```python
from build123d import *

# Parameters (mm, degrees)
F0_W     = 85
F0_H     = 56
F0_R     = 1.375
F1_DEPTH = 1.5
F2_W     = 14.5066131875
F2_H     = 7.0550842881
F2_H_2   = 1.0795340971
F3_DEPTH = 4
F2_W_2   = 52.5494457505
F2_H_3   = 3.6331438509
F4_DEPTH = 9
F2_W_3   = 0.706913475
F2_H_4   = 12.0032178172
F2_W_4   = 17.4915134945
F2_W_5   = 0.87367237
F2_W_6   = 17.3247545996
F5_DEPTH = 15
F2_W_7   = 20.1837714718
F2_H_5   = 16.9899400229
F2_W_8   = 1.3980423616
F6_DEPTH = 13


with BuildPart() as f1:
    # F0 (on Top) → F1 (new body)
    with BuildSketch(Plane.XY):
        Rectangle(F0_W, F0_H)
        with Locations((-39, -24.5)):
            Circle(F0_R, mode=Mode.SUBTRACT)
        with Locations((19, -24.5)):
            Circle(F0_R, mode=Mode.SUBTRACT)
        with Locations((-39, 24.5)):
            Circle(F0_R, mode=Mode.SUBTRACT)
        with Locations((19, 24.5)):
            Circle(F0_R, mode=Mode.SUBTRACT)
    extrude(amount=F1_DEPTH)

    # F2 (on face) → F3 (join)
    with BuildSketch(Plane.XY.offset(1.5)):
        with Locations((-10.5, -24.4724578559)):
            Rectangle(F2_W, F2_H)
        with Locations((-10.5, -28.5397670486)):
            Rectangle(F2_W, F2_H_2)
    extrude(amount=F3_DEPTH)

    # F2 (on face) → F4 (join)
    with BuildSketch(Plane.XY.offset(1.5)):
        with Locations((-9.9811840151, 23.979865989)):
            Rectangle(F2_W_2, F2_H_3)
    extrude(amount=F4_DEPTH)

    # F2 (on face) → F5 (join)
    with BuildSketch(Plane.XY.offset(1.5)):
        with Locations((42.8534567375, 3.2353831921)):
            Rectangle(F2_W_3, F2_H_4)
        with Locations((33.7542432528, 3.2353831921)):
            Rectangle(F2_W_4, F2_H_4)
        with Locations((42.936836185, 19.5779297501)):
            Rectangle(F2_W_5, F2_H_4)
        with Locations((33.8376227002, 19.5779297501)):
            Rectangle(F2_W_6, F2_H_4)
    extrude(amount=F5_DEPTH)

    # F2 (on face) → F6 (join)
    with BuildSketch(Plane.XY.offset(1.5)):
        with Locations((32.4081142641, -15.4418135062)):
            Rectangle(F2_W_7, F2_H_5)
        with Locations((43.1990211808, -15.4418135062)):
            Rectangle(F2_W_8, F2_H_5)
    extrude(amount=F6_DEPTH)


solid = f1.part
```
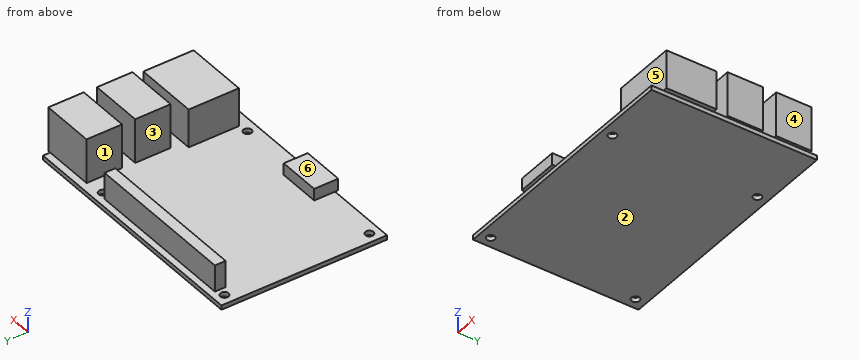
Part model, mm, in its own coordinate system. Face numbers are marked on the shaded views. A direction names the side the tool comes from. Give positions to 0.01 mm unless a question says otherwise; leave off trailing zeros. Order: outer loops, then holes, each group sorted by start corner. A loop starts at its lowest first (then second) coordinate and runs counter-clockwise, first axis right, second up. Notation, with made-up numbers: M 84.5,42 L 126.5,42 A28 ccw 126.5,73 Z; hole C 81.5,87 d8. An arc over 180 degrees is marked long. Use a Markdown table: item, result. Add a question column.
(1) Probe line 1 along Y through (x, z) = (19, 0.55) (3 decimals); line 2 along Y through (x, z) = (25.5, 11.5); line 3 along X through (y, z) = (25.5, 10). List the from-to ranges inside material, lowest first. Write a range as [from, to].
(2) Saw through at B-B, the plane z = 12.25. Give the cut face in (x, y).
(3) Saw through at C-C, the plane x = 19. Give the cut face in (y, z) (3 decimals).
(4) Saw through at D-D, the plane z = 3.25. Give the cut face in (x, y).
(5) 3-axis set-ups, long thin cutter, end or side, ignore diameter. For the marked faces 4, 5 and 6: which of +Z, -Z, +X, -X, +Y, -Y reach the whole face in a straight line?
(6) Drop flat-ended pins along their axis: P1, Ø1.2, axis at y = -4.5, z = 1, coming from the +X side; P2, Ø3, axis at y = 24.5, z = 8, coming from the -X side; P3, Ø3.5, axis at x = 19, y = -24.5, coming from the +Z side; P4, Ø2.5, axis at x = -13, z = 6.5, coming from the -Y side. Give the stop position or say it passes through.
(7) Mould opens along X. For the marked faces 1, 2 and 3 say: +X half, -X half, draft (parallel to the pull), parting line (faces both ways), or undercut.
(8) Saw through at A-A, the plane y = 24.5. Give the cut face in (x, z) (3 decimals).
Answer key:
| question | item | result |
|---|---|---|
| 1 | line 1 | [-28, -25.875], [-23.125, 23.125], [25.875, 28] |
| 1 | line 2 | [-23.94, -6.95], [-2.77, 9.24], [13.58, 25.58] |
| 1 | line 3 | [-36.26, 16.29], [25.18, 43.37] |
| 2 | outline | M 22.32,-23.94 L 43.9,-23.94 L 43.9,-6.95 L 22.32,-6.95 Z; M 25.01,-2.77 L 43.21,-2.77 L 43.21,9.24 L 25.01,9.24 Z; M 25.18,13.58 L 43.37,13.58 L 43.37,25.58 L 25.18,25.58 Z |
| 3 | outline | M -28,0 L -25.875,0 L -25.875,1.5 L -28,1.5 Z; M -23.125,0 L 23.125,0 L 23.125,1.5 L -23.125,1.5 Z; M 25.875,0 L 28,0 L 28,1.5 L 25.875,1.5 Z |
| 4 | outline | M -36.26,22.16 L 16.29,22.16 L 16.29,25.8 L -36.26,25.8 Z; M -17.75,-29.08 L -3.25,-29.08 L -3.25,-20.94 L -17.75,-20.94 Z; M 22.32,-23.94 L 43.9,-23.94 L 43.9,-6.95 L 22.32,-6.95 Z; M 25.01,-2.77 L 43.21,-2.77 L 43.21,9.24 L 25.01,9.24 Z; M 25.18,13.58 L 43.37,13.58 L 43.37,25.58 L 25.18,25.58 Z |
| 5 | face 4 | +Z, -Z, +X, +Y |
| 5 | face 5 | +Z, +X, -Y |
| 5 | face 6 | +Z, -X, -Y |
| 6 | P1 | x = 42.5 |
| 6 | P2 | x = -36.26 |
| 6 | P3 | z = 1.5 |
| 6 | P4 | y = -29.08 |
| 7 | face 1 | undercut |
| 7 | face 2 | draft |
| 7 | face 3 | -X half |
| 8 | outline | M -42.5,0 L -40.375,0 L -40.375,1.5 L -42.5,1.5 Z; M -37.625,0 L 17.625,0 L 17.625,1.5 L 16.294,1.5 L 16.294,10.5 L -36.256,10.5 L -36.256,1.5 L -37.625,1.5 Z; M 20.375,0 L 42.5,0 L 42.5,1.5 L 43.374,1.5 L 43.374,16.5 L 25.175,16.5 L 25.175,1.5 L 20.375,1.5 Z |
